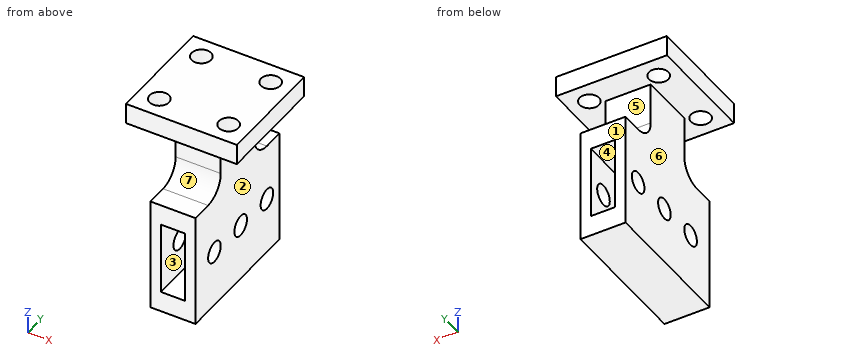
from build123d import *

# Parameters (mm, degrees)
SKETCH1_W           = 6.5
SKETCH1_H           = 25.5
SKETCH1_W_2         = 3.5
SKETCH1_H_2         = 10.5
BOSS_EXTRUDE1_DEPTH = 10
SKETCH2_W           = 16
SKETCH2_H           = 3
BOSS_EXTRUDE2_DEPTH = 8
CUT_EXTRUDE1_REACH  = 23.786
CUT_EXTRUDE2_REACH  = 33.245
SKETCH4_R           = 1.4
FILLET1_R           = 3
SKETCH6_R           = 1.5
CUT_EXTRUDE4_DEPTH  = 22.785889929


with BuildPart() as part:
    # Sketch1 → Boss-Extrude1 (new, symmetric)
    with BuildSketch(Plane(origin=(0, 0, 0), x_dir=(1, 0, 0), z_dir=(0, 1, 0))):
        Rectangle(SKETCH1_W, SKETCH1_H)
        with Locations((0, 4.5)):
            Rectangle(SKETCH1_W_2, SKETCH1_H_2, mode=Mode.SUBTRACT)
    extrude(amount=BOSS_EXTRUDE1_DEPTH, both=True)

    # Sketch2 → Boss-Extrude2 (add, symmetric)
    with BuildSketch(Plane.XZ):
        with Locations((0, 14.25)):
            Rectangle(SKETCH2_W, SKETCH2_H)
    extrude(amount=BOSS_EXTRUDE2_DEPTH, both=True)

    # Sketch3 → Cut-Extrude1 (cut, up to next)
    with BuildSketch(Plane.ZY.offset(3.25), mode=Mode.PRIVATE) as cut_extrude1_sk1:
        Polygon((12.75, -4), (3.75, -4), (3.75, -10), (12.75, -10), (12.75, -8), align=None)
    cut_extrude1_tool1 = extrude(cut_extrude1_sk1.sketch, amount=-CUT_EXTRUDE1_REACH, mode=Mode.PRIVATE) & part.part
    # Sketch3 → Cut-Extrude1 (cut, up to next)
    with BuildSketch(Plane.ZY.offset(3.25), mode=Mode.PRIVATE) as cut_extrude1_sk2:
        Polygon((12.75, 8), (12.75, 10), (3.75, 10), (3.75, 4), (12.75, 4), align=None)
    cut_extrude1_tool2 = extrude(cut_extrude1_sk2.sketch, amount=-CUT_EXTRUDE1_REACH, mode=Mode.PRIVATE) & part.part
    add(cut_extrude1_tool1.solids().sort_by_distance((-3.25, -7, 8.25))[0], mode=Mode.SUBTRACT)
    add(cut_extrude1_tool2.solids().sort_by_distance((-3.25, 7, 8.25))[0], mode=Mode.SUBTRACT)

    # Sketch4 → Cut-Extrude2 (cut, up to next)
    with BuildSketch(Plane.XY.offset(15.75), mode=Mode.PRIVATE) as cut_extrude2_sk1:
        with Locations((5, -5)):
            Circle(SKETCH4_R)
    cut_extrude2_tool1 = extrude(cut_extrude2_sk1.sketch, amount=-CUT_EXTRUDE2_REACH, mode=Mode.PRIVATE) & part.part
    # Sketch4 → Cut-Extrude2 (cut, up to next)
    with BuildSketch(Plane.XY.offset(15.75), mode=Mode.PRIVATE) as cut_extrude2_sk2:
        with Locations((5, 5)):
            Circle(SKETCH4_R)
    cut_extrude2_tool2 = extrude(cut_extrude2_sk2.sketch, amount=-CUT_EXTRUDE2_REACH, mode=Mode.PRIVATE) & part.part
    # Sketch4 → Cut-Extrude2 (cut, up to next)
    with BuildSketch(Plane.XY.offset(15.75), mode=Mode.PRIVATE) as cut_extrude2_sk3:
        with Locations((-5, 5)):
            Circle(SKETCH4_R)
    cut_extrude2_tool3 = extrude(cut_extrude2_sk3.sketch, amount=-CUT_EXTRUDE2_REACH, mode=Mode.PRIVATE) & part.part
    # Sketch4 → Cut-Extrude2 (cut, up to next)
    with BuildSketch(Plane.XY.offset(15.75), mode=Mode.PRIVATE) as cut_extrude2_sk4:
        with Locations((-5, -5)):
            Circle(SKETCH4_R)
    cut_extrude2_tool4 = extrude(cut_extrude2_sk4.sketch, amount=-CUT_EXTRUDE2_REACH, mode=Mode.PRIVATE) & part.part
    add(cut_extrude2_tool1.solids().sort_by_distance((5, -5, 15.75))[0], mode=Mode.SUBTRACT)
    add(cut_extrude2_tool2.solids().sort_by_distance((5, 5, 15.75))[0], mode=Mode.SUBTRACT)
    add(cut_extrude2_tool3.solids().sort_by_distance((-5, 5, 15.75))[0], mode=Mode.SUBTRACT)
    add(cut_extrude2_tool4.solids().sort_by_distance((-5, -5, 15.75))[0], mode=Mode.SUBTRACT)

    # Fillet1
    fillet1_edges = [part.edges().sort_by_distance(p)[0] for p in [
        (0, -4, 3.75),
        (0, 4, 3.75),
    ]]
    fillet(fillet1_edges, radius=FILLET1_R)

    # Sketch6 → Cut-Extrude4 (cut, through all)
    with BuildSketch(Plane(origin=(3.25, 0, 0), x_dir=(0, 0, -1), z_dir=(1, 0, 0))):
        with Locations((4.5, 7)):
            Circle(SKETCH6_R)
        with Locations((4.5, -5.5)):
            Circle(SKETCH6_R)
        with Locations((4.5, 0.75)):
            Circle(SKETCH6_R)
    extrude(amount=-CUT_EXTRUDE4_DEPTH, mode=Mode.SUBTRACT)


solid = part.part
Could you check a few things on this model? Use its own coordinates, in mm. Face numbers are marked on the shaded views. A direction names the side the tool comes from. Give positions to 0.01 mm unless a question says otherwise; leave off trailing zeros. Order: outer loops, then holes, each group sorted by start corner. A loop starts at its lowest first (then second) coordinate and runs counter-clockwise, first axis right, second up. Notation, with made-up numbers: (-37.5, -23.5) - (2.5, -23.5) arc R20 ccw to (2.5, 1.5) - close; hole circle Ø9 at (-23.5, 28). An arc over 180 degrees is marked (long way). One line per question, with ' | ' between items. Start each with the question number.
Item 1: Thinking about a two-plate mould opening in X: for the marked faces 1, 2 and 3, which applies, pulls with the +X half, pulls with the -X half, needs draft (parallel to the pull), parting line crosses it, or undercut?
Item 2: I want a section at B-B on x = -2.75. Write out the boundary of the cut face in (y, z).
Item 3: I want a section at A-A on y = -7.5. Write out the boundary of the cut face in (x, z).
Item 4: I want a section at D-D on z = -8.25. Write out the boundary of the cut face in (x, y), then the cut area to 3 significant figures.
Item 5: I'm going to push flat-ended pins straight in: pin 1 Ø3 at (x, y) = (5, -5) entering from -Z; pin 2 Ø5 at (x, z) = (-1, 9.5) entering from -Y; pin 3 Ø10 at (y, z) = (2.5, 3.5) entering from -X. Where does each tip first touch, or does it pass through?
Item 6: For the marked faces 4, 5, 6 and 7, which set-ups out of +Z, -Z, +X, -X, +Y, -Y let a thin tool reach every point of the face, with its end or its side?
Item 7: I need wall thicknesses on probe 1 along Y at (x, z) = (5, 13.8); probe 2 along X at (y, z) = (5, -5); probe 3 along Z at (x, y) = (-2.75, -6.5). Which ranges of each line are inside material? Lowest first, please. Write a range as [from, to].
Item 8: I want a section at C-C on y = 0.75. Write out the boundary of the cut face in (x, z), then the cut area to 3 significant figures.
Verdict:
1) face 1: needs draft | face 2: pulls with the +X half | face 3: undercut
2) outline: (-10, -12.75) - (10, -12.75) - (10, 3.75) - (7, 3.75) arc R3 cw to (4, 6.75) - (4, 12.75) - (8, 12.75) - (8, 15.75) - (-8, 15.75) - (-8, 12.75) - (-4, 12.75) - (-4, 6.75) arc R3 cw to (-7, 3.75) - (-10, 3.75) - close; hole circle Ø3 at (-5.5, -4.5); hole circle Ø3 at (0.75, -4.5); hole circle Ø3 at (7, -4.5)
3) outline: (-8, 12.75) - (8, 12.75) - (8, 15.75) - (-8, 15.75) - close; (-3.25, -12.75) - (3.25, -12.75) - (3.25, 3.75) - (-3.25, 3.75) - close; hole (-1.75, -9.75) - (1.75, -9.75) - (1.75, 0.75) - (-1.75, 0.75) - close
4) outline: (-3.25, -10) - (-1.75, -10) - (-1.75, 10) - (-3.25, 10) - close; (1.75, -10) - (3.25, -10) - (3.25, 10) - (1.75, 10) - close | area: 60.0 mm^2
5) pin 1: z = 12.75 | pin 2: y = -4 | pin 3: x = -3.25
6) face 4: +Y, -Y | face 5: +X, -X, +Y | face 6: -Z, -X, +Y, -Y | face 7: +X, -X, -Y
7) probe 1: [-8, -6.4], [-3.6, 3.6], [6.4, 8] | probe 2: [-3.25, -1.75], [1.75, 3.25] | probe 3: [-12.75, -5.62], [-3.38, 3.79], [12.75, 15.75]
8) outline: (-8, 12.75) - (-3.25, 12.75) - (-3.25, -3) - (-1.75, -3) - (-1.75, 0.75) - (1.75, 0.75) - (1.75, -3) - (3.25, -3) - (3.25, 12.75) - (8, 12.75) - (8, 15.75) - (-8, 15.75) - close; (-3.25, -12.75) - (3.25, -12.75) - (3.25, -6) - (1.75, -6) - (1.75, -9.75) - (-1.75, -9.75) - (-1.75, -6) - (-3.25, -6) - close | area: 168 mm^2
